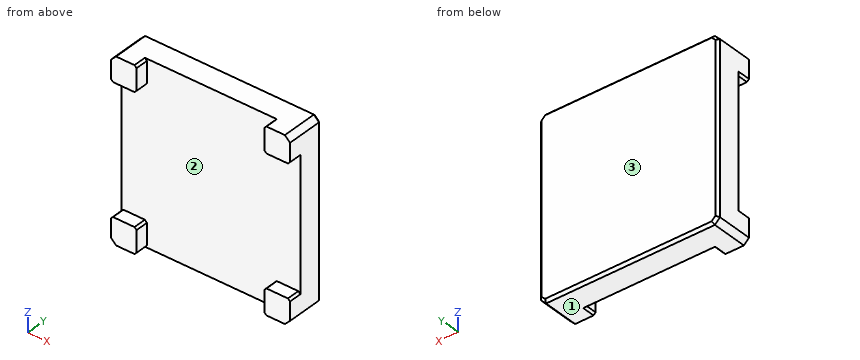
```python
from build123d import *

# Parameters (mm, degrees)
SKETCH1_W           = 88.9
SKETCH1_H           = 88.9
BOSS_EXTRUDE1_DEPTH = 19.05
CUT_EXTRUDE1_DEPTH  = 6.35
LEGS_OUTER_SIZE     = 2.54
TOP_FACE_SIZE       = 1.27
LEGS_INNER_SIZE     = 1.016


with BuildPart() as part:
    # Sketch1 → Boss-Extrude1 (new body)
    with BuildSketch(Plane(origin=(0, 0, 0), x_dir=(1, 0, 0), z_dir=(0, 1, 0))):
        Rectangle(SKETCH1_W, SKETCH1_H)
    extrude(amount=BOSS_EXTRUDE1_DEPTH)

    # Sketch1<3> → Cut-Extrude1 (cut)
    with BuildSketch(Plane(origin=(0, 0, 0), x_dir=(1, 0, 0), z_dir=(0, 1, 0))):
        Polygon((-44.45, -31.75), (-31.75, -31.75), (-31.75, -44.45), (31.75, -44.45), (31.75, -31.75), (44.45, -31.75), (44.45, 31.75), (31.75, 31.75), (31.75, 44.45), (-31.75, 44.45), (-31.75, 31.75), (-44.45, 31.75), align=None)
    extrude(amount=CUT_EXTRUDE1_DEPTH, mode=Mode.SUBTRACT)

    # legs, outer
    legs_outer_edges = [part.edges().sort_by_distance(p)[0] for p in [
        (-44.45, 9.525, 44.45),
        (44.45, 9.525, 44.45),
        (44.45, 9.525, -44.45),
        (-44.45, 9.525, -44.45),
    ]]
    chamfer(legs_outer_edges, length=LEGS_OUTER_SIZE)

    # top face
    top_face_edges = [part.edges().sort_by_distance(p)[0] for p in [
        (0, 19.05, -44.45),
        (44.45, 19.05, 0),
        (-44.45, 19.05, 0),
        (0, 19.05, 44.45),
        (-43.18, 19.05, -43.18),
        (-43.18, 19.05, 43.18),
        (43.18, 19.05, 43.18),
        (43.18, 19.05, -43.18),
    ]]
    chamfer(top_face_edges, length=TOP_FACE_SIZE)

    # legs, inner
    legs_inner_edges = [part.edges().sort_by_distance(p)[0] for p in [
        (-44.45, 3.175, 31.75),
        (-44.45, 3.175, -31.75),
        (-31.75, 3.175, -31.75),
        (-31.75, 3.175, -44.45),
        (31.75, 3.175, -44.45),
        (31.75, 3.175, -31.75),
        (44.45, 3.175, -31.75),
        (44.45, 3.175, 31.75),
        (31.75, 3.175, 31.75),
        (31.75, 3.175, 44.45),
        (-31.75, 3.175, 44.45),
        (-31.75, 3.175, 31.75),
    ]]
    chamfer(legs_inner_edges, length=LEGS_INNER_SIZE)


solid = part.part
```
CAD build for the part. Positions are in the model's coordinates, mm. Face numbers are marked on the shaded views. Round coordinates to 2 decimals unless told otherwise and drop trailing zeros. Loops run counter-clockwise (first coordinate to the right, second up) from the corner with the lowest first, then second, coordinate; pieces in that order, holes last. Notation, with made-up numbers: M -36.5,-34 L -6.5,-34 A24 ccw -6.5,-14 Z; hole C 2.5,-27 d7. An arc over 180 degrees is marked long. Use a Markdown table: item, result. Add a question column.
(1) Cut at D-D (z = 36.5). Give the cut face in (x, y), and give its area (3 significant figures).
(2) Flat gauge pin, fed straight in: pin 1 (1 mm diameter, centred on x = -31.5, z = -18.5, fed in from -Y). Where does the tip first touch, or does it go through?
(3) Pull direction Z, two halves, no side cores. Call the marked faces 1, 2 and 3: +Z half, -Z half, draft (parallel to the pull), parting line (faces both ways), or undercut.
(4) Drill centre lines: line 1 (Z direction, x = -38.5, y = 1.5); line 2 (Y direction, x = 13, z = -2); line 3 (Z direction, x = -32.5, y = 3). Where is each one in solid material? Low to high.
(5) Cut at B-B (z = 16). Give the cut face in (x, y).
(6) Cut at A-A (y = 2.5). State how many separate pieces and enclosed holes the cut face has, and give its area (3 significant figures).
(7) Cut at C-C (x = -3.5). Give the cut face in (y, z), and give its area (3 significant figures).
Geometry says:
| question | item | result |
|---|---|---|
| 1 | outline | M -44.45,0 L -31.75,0 L -31.75,6.35 L 31.75,6.35 L 31.75,0 L 44.45,0 L 44.45,17.78 L 43.18,19.05 L -43.18,19.05 L -44.45,17.78 Z |
| 1 | area | 1,290 mm² |
| 2 | pin 1 | stops at y = 6.35 |
| 3 | face 1 | -Z half |
| 3 | face 2 | undercut |
| 3 | face 3 | draft |
| 4 | line 1 | z = -44.45 to -31.75, 31.75 to 44.45 |
| 4 | line 2 | y = 6.35 to 19.05 |
| 4 | line 3 | z = -44.18 to -32.02, 32.02 to 44.18 |
| 5 | outline | M -44.45,6.35 L 44.45,6.35 L 44.45,17.78 L 43.18,19.05 L -43.18,19.05 L -44.45,17.78 Z |
| 6 | separate pieces | 4 |
| 6 | enclosed holes | 0 |
| 6 | area | 626 mm² |
| 7 | outline | M 6.35,-44.45 L 17.78,-44.45 L 19.05,-43.18 L 19.05,43.18 L 17.78,44.45 L 6.35,44.45 Z |
| 7 | area | 1,130 mm² |
